Check sheet for the modelled part. Datum: model origin and axes. Units: mm. A direction names the side the tool comes from. Coordinates: 2 decimals unless noted, no trailing zeros. Write each loop counter-clockwise with the first axis right and the second up, starting at its lowest first coordinate (ties: lowest second). Pieces come first, ordered by that corner, then holes. Notation, with made-up numbers: (-27.75, 72.25) -> (29.25, 72.25) arc R13 cw to (29.25, 89.25) -> close; hole circle Ø5 at (-24.5, 18.5). An arc over 180 degrees is marked (long way). One line per item, written item: value. Start each with the question number.
1) Sectioned sample at B-B on y = 6. Enter the section's corners in (x, z), plus the area to 3 significant figures.
2) Gauge pin test, flat ends, axial feed: P1, Ø1.7, axis at x = -13.6, y = 19.26, coming from the +Z side; P2, Ø1.5, axis at y = 21.5, z = 3.5, coming from the -X side; P3, Ø8, axis at y = 16, z = 3, coming from the -X side. Record the tip position at first contact, or that the pin passes through.
3) Sectioned sample at D-D on x = 26. Enter the section's corners in (y, z).
4) Set-up check for faces 4 (the cylindrical face through (20.723, 28.746, 8.67)), 5 (the flat face through (4.81, 22.28, 1.48)): record each of +Z, -Z, +X, -X, +Y, -Y from which the full face is reachable in a straight line by a thin tool's end or side.
5) Sectioned sample at C-C on z = 4.5. Give the number of separate pieces and of enclosed holes in the cut face, plus the area to 3 significant figures.
6) Sectioned sample at A-A on x = -7.5. Enter the section's corners in (y, z).
7) Scan lines: line 1 along X through (y, z) = (30, 9.75); line 2 along Y through (x, z) = (-13, 13.25); line 3 along Y through (x, z) = (17.5, 12.75). Record each from-to range of solid material in increasing order. Write a range as [from, to].
8) Draft check along X on faces 1 (the flat face through (21.61, 7.08, 1.48)), 2 (the flat face through (-2.744, 2.805, 1.479)), 3 (the flat face through (16.56, 12.8, 1.48)). Enter one of: +X half, -X half, draft (parallel to the pull), parting line (faces both ways), or undercut.
```python
from build123d import *

# Parameters (mm, degrees)
F0_R        = 1.75
F1_DEPTH    = 3
F0_R_2      = 1.4
F2_DEPTH    = 14.5
F3_DEPTH    = 3
F4_R        = 7
F5_T1_DEPTH = 16.6306186867
F5_T3_DEPTH = 4.3681636199
F5_T5_DEPTH = 16.0958411758
F7_DEPTH    = 3


# Not quite as in the source:
# - a fillet or chamfer that OpenCascade refuses, or shapes differently, is made with other operations: its cross-section is extruded or revolved along the edge and cut away or added
# - two fillets or chamfers of one size are made in one step


with BuildPart() as f1:
    # F0 (on Top) → F1 (new body)
    with BuildSketch(Plane.XY):
        with BuildLine():
            Line((-0.4909088138, -1.2505585665), (20.7660850672, -2.35005825))
            Line((20.7660850672, -2.35005825), (25.5381567791, -2.5968895454))
            ThreePointArc((25.5381567791, -2.5968895454), (27.0513379129, -0.9141469555), (27.3799938245, 1.3248986134))
            Line((27.3799938245, 1.3248986134), (27.2720971653, 1.8240689049))
            Line((27.2720971653, 1.8240689049), (21.7261834625, 27.4815394929))
            ThreePointArc((21.7261834625, 27.4815394929), (17.3096816882, 28.8299287619), (19.4503780507, 32.9215128838))
            Line((19.4503780507, 32.9215128838), (18.5115177807, 34.0451927012))
            Line((18.5115177807, 34.0451927012), (15.1742594532, 34.2144082882))
            Line((15.1742594532, 34.2144082882), (15.9797014768, 30.8189948872))
            Line((15.9797014768, 30.8189948872), (16.4916617939, 28.6607800556))
            Line((16.4916617939, 28.6607800556), (18.135858017, 21.7295227758))
            Line((18.135858017, 21.7295227758), (18.644845427, 19.5838405017))
            Line((18.644845427, 19.5838405017), (20.2910235881, 12.6442281836))
            Line((20.2910235881, 12.6442281836), (20.8000109982, 10.4985459094))
            Line((20.8000109982, 10.4985459094), (22.4442072213, 3.5672886297))
            Line((22.4442072213, 3.5672886297), (14.8716080252, 3.8805312748))
            Line((14.8716080252, 3.8805312748), (12.8516365903, 3.9640879479))
            Line((12.8516365903, 3.9640879479), (5.2790373942, 4.2773305929))
            Line((5.2790373942, 4.2773305929), (3.2590659592, 4.360887266))
            Line((3.2590659592, 4.360887266), (0, 4.4956994243))
            Line((0, 4.4956994243), (-4.5071129665, 11.5453820412))
            Line((-4.5071129665, 11.5453820412), (-5.9023623433, 13.727724785))
            Line((-5.9023623433, 13.727724785), (-6.7908302355, 15.1173985523))
            Line((-6.7908302355, 15.1173985523), (-9.9708875905, 20.0914019161))
            Line((-9.9708875905, 20.0914019161), (-10.4149082493, 20.7859051919))
            Line((-10.4149082493, 20.7859051919), (-11.8101576261, 22.9682479357))
            Line((-11.8101576261, 22.9682479357), (-12.6478674294, 24.2785297685))
            Line((-12.6478674294, 24.2785297685), (-13.4783331305, 23.2781674713))
            Line((-13.4783331305, 23.2781674713), (-11.5363753254, 21.4427254814))
            ThreePointArc((-11.5363753254, 21.4427254814), (-12.0316990994, 16.7032264224), (-16.4766345607, 18.4209998989))
            Line((-16.4766345607, 18.4209998989), (-15.4909088138, 7.2494414335))
            Line((-15.4909088138, 7.2494414335), (-4.9353532582, 6.7494414335))
            Line((-4.9353532582, 6.7494414335), (-0.4909088138, -1.2505585665))
        make_face()
        with Locations((23.5090911862, 0.7494414335)):
            Circle(F0_R, mode=Mode.SUBTRACT)
    extrude(amount=F1_DEPTH)

    # F0 (on Top) → F2 (join)
    with BuildSketch(Plane.XY):
        with BuildLine():
            Line((-16.9909088138, 24.2494414335), (-16.4766345607, 18.4209998989))
            ThreePointArc((-16.4766345607, 18.4209998989), (-12.0316990994, 16.7032264224), (-11.5363753254, 21.4427254814))
            Line((-11.5363753254, 21.4427254814), (-13.4783331305, 23.2781674713))
            Line((-13.4783331305, 23.2781674713), (-12.6478674294, 24.2785297685))
            Line((-12.6478674294, 24.2785297685), (-11.3383288336, 25.8559736489))
            Line((-11.3383288336, 25.8559736489), (-9.782692223, 27.729862253))
            Line((-9.782692223, 27.729862253), (-8.1632279798, 29.680636341))
            Line((-8.1632279798, 29.680636341), (-6.4480341787, 31.746724331))
            Line((-6.4480341787, 31.746724331), (-4.9677388347, 33.5298583591))
            ThreePointArc((-4.9677388347, 33.5298583591), (-4.3296328325, 33.596636032), (-3.691225205, 33.6604657178))
            ThreePointArc((-3.691225205, 33.6604657178), (-2.7124843131, 33.7525453098), (-1.7331162834, 33.8376960422))
            ThreePointArc((-1.7331162834, 33.8376960422), (1.9635943301, 34.0963274062), (5.6658885292, 34.2562561568))
            ThreePointArc((5.6658885292, 34.2562561568), (6.6605332405, 34.2823712951), (7.6553394943, 34.3013612736))
            ThreePointArc((7.6553394943, 34.3013612736), (11.4153879508, 34.3087710358), (15.1742594532, 34.2144082882))
            Line((15.1742594532, 34.2144082882), (18.5115177807, 34.0451927012))
            Line((18.5115177807, 34.0451927012), (19.4503780507, 32.9215128838))
            ThreePointArc((19.4503780507, 32.9215128838), (17.3096816882, 28.8299287619), (21.7261834625, 27.4815394929))
            Line((21.7261834625, 27.4815394929), (21.7201782041, 27.5093220636))
            Line((21.7201782041, 27.5093220636), (28.8304557098, 35.6590934098))
            ThreePointArc((28.8304557098, 35.6590934098), (10.8304557098, 36.6599030898), (-7.1695442902, 35.6590934098))
            Line((-7.1695442902, 35.6590934098), (-16.9909088138, 24.2494414335))
        make_face()
        with Locations((-13.5970591864, 19.2624543916)):
            Circle(F0_R_2, mode=Mode.SUBTRACT)
        with Locations((20.077256969, 29.9877400872)):
            Circle(F0_R_2, mode=Mode.SUBTRACT)
    extrude(amount=F2_DEPTH)

    # F0 (on Top) → F3 (join)
    with BuildSketch(Plane.XY):
        with BuildLine():
            Line((-9.782692223, 27.729862253), (-11.3383288336, 25.8559736489))
            Line((-11.3383288336, 25.8559736489), (-10.6418538761, 22.9199207303))
            Line((-10.6418538761, 22.9199207303), (-11.8101576261, 22.9682479357))
            Line((-11.8101576261, 22.9682479357), (-10.4149082493, 20.7859051919))
            Line((-10.4149082493, 20.7859051919), (-10.132866466, 20.7742384561))
            Line((-10.132866466, 20.7742384561), (-9.9708875905, 20.0914019161))
            Line((-9.9708875905, 20.0914019161), (-6.7908302355, 15.1173985523))
            Line((-6.7908302355, 15.1173985523), (-8.112895031, 20.690681783))
            Line((-8.112895031, 20.690681783), (-0.540295835, 20.3774391379))
            Line((-0.540295835, 20.377439138), (1.1058823261, 13.4378268199))
            Line((1.1058823261, 13.4378268199), (-5.9023623433, 13.727724785))
            Line((-5.9023623433, 13.727724785), (-4.5071129665, 11.5453820412))
            Line((-4.5071129665, 11.5453820412), (1.6148697362, 11.2921445457))
            Line((1.6148697362, 11.2921445457), (3.2590659592, 4.360887266))
            Line((3.2590659592, 4.360887266), (5.2790373942, 4.2773305929))
            Line((5.2790373942, 4.2773305929), (3.6348411711, 11.2085878727))
            Line((3.6348411711, 11.2085878727), (11.2074403672, 10.8953452276))
            Line((11.2074403672, 10.8953452276), (12.8516365903, 3.9640879479))
            Line((12.8516365903, 3.9640879479), (14.8716080252, 3.8805312748))
            Line((14.8716080252, 3.8805312748), (13.2274118021, 10.8117885545))
            Line((13.2274118021, 10.8117885545), (20.8000109982, 10.4985459094))
            Line((20.8000109982, 10.4985459094), (20.2910235881, 12.6442281836))
            Line((20.2910235881, 12.6442281836), (12.7184243921, 12.9574708287))
            Line((12.7184243921, 12.9574708287), (11.072246231, 19.8970831467))
            Line((11.072246231, 19.8970831467), (18.644845427, 19.5838405017))
            Line((18.644845427, 19.5838405017), (18.135858017, 21.7295227758))
            Line((18.135858017, 21.7295227758), (10.5632588209, 22.0427654209))
            Line((10.5632588209, 22.0427654209), (8.9190625979, 28.9740227006))
            Line((8.9190625979, 28.9740227006), (16.4916617939, 28.6607800556))
            Line((16.4916617939, 28.6607800556), (15.9797014768, 30.8189948872))
            Line((15.9797014768, 30.8189948872), (8.4071022808, 31.1322375323))
            Line((8.4071022808, 31.1322375323), (7.6553394943, 34.3013612736))
            ThreePointArc((7.6553394943, 34.3013612736), (6.6605332405, 34.2823712951), (5.6658885292, 34.2562561568))
            Line((5.6658885292, 34.2562561568), (6.3871308458, 31.2157942054))
            Line((6.3871308458, 31.2157942054), (-1.1854683502, 31.5290368504))
            Line((-1.1854683502, 31.5290368504), (-1.7331162834, 33.8376960422))
            ThreePointArc((-1.7331162834, 33.8376960422), (-2.7124843131, 33.7525453098), (-3.691225205, 33.6604657178))
            Line((-3.691225205, 33.6604657178), (-3.2054397853, 31.6125935235))
            Line((-3.2054397853, 31.6125935235), (-6.4480341787, 31.746724331))
            Line((-6.4480341787, 31.746724331), (-8.1632279798, 29.680636341))
            Line((-8.1632279798, 29.680636341), (-2.6934794682, 29.4543786918))
            Line((-2.6934794682, 29.4543786918), (-1.0492832451, 22.5231214121))
            Line((-1.0492832451, 22.5231214121), (-8.6218824411, 22.8363640572))
            Line((-8.6218824411, 22.8363640572), (-9.782692223, 27.729862253))
        make_face()
        Polygon((1.4796756, 20.2938824649), (9.052274796, 19.9806398198), (10.6984529571, 13.0410275017), (3.1258537611, 13.3542701468), align=None, mode=Mode.SUBTRACT)
        Polygon((8.543287386, 22.126322094), (0.9706881899, 22.439564739), (-0.6735080331, 29.3708220188), (6.8990911629, 29.0575793737), align=None, mode=Mode.SUBTRACT)
    extrude(amount=F3_DEPTH)

    # F4
    f4_edges = [f1.edges().sort_by_distance(p)[0] for p in [
        (-7.169544, 35.659093, 7.25),
    ]]
    fillet(f4_edges, radius=F4_R)

    # F5: fillet of radius 3 on 3 edges, made by hand

    # F5_s2 → F5_t1 (cut)
    with BuildSketch(Plane.XY.offset(-6.8153093434)):
        with BuildLine():
            ThreePointArc((27.2309502901, -0.4600225022), (26.0778302758, -2.0046934728), (24.2228512202, -2.5288564993))
            Line((24.2228512202, -2.5288564993), (25.5381567791, -2.5968895454))
            ThreePointArc((25.5381567791, -2.5968895454), (26.5766364437, -1.6806211776), (27.2309502901, -0.4600225022))
        make_face()
    extrude(amount=F5_T1_DEPTH, mode=Mode.SUBTRACT)

    # F5_s4 → F5_t3 (cut)
    with BuildSketch(Plane.XY.offset(-0.6840818099)):
        with BuildLine():
            ThreePointArc((27.3520636944, 1.4541138391), (27.3881865873, 1.2545487843), (27.4107435182, 1.0529991394))
            ThreePointArc((27.4107435182, 1.0529991394), (27.3977458408, 1.1892177156), (27.3799938245, 1.3248986134))
            Line((27.3799938245, 1.3248986134), (27.3520636944, 1.4541138391))
        make_face()
    extrude(amount=F5_T3_DEPTH, mode=Mode.SUBTRACT)

    # F5_s6 → F5_t5 (cut)
    with BuildSketch(Plane.XY.offset(-6.5479205879)):
        with BuildLine():
            ThreePointArc((-15.7211174898, 9.8584730948), (-14.8104709381, 7.9581341855), (-12.8746740451, 7.1255145234))
            Line((-12.8746740451, 7.1255145234), (-15.4909088138, 7.2494414335))
            Line((-15.4909088138, 7.2494414335), (-15.7211174898, 9.8584730948))
        make_face()
    extrude(amount=F5_T5_DEPTH, mode=Mode.SUBTRACT)

    # F0 (on Top) → F7 (join)
    with BuildSketch(Plane.XY):
        with Locations((20.077256969, 29.9877400872)):
            Circle(F0_R_2)
        with Locations((-13.5970591864, 19.2624543916)):
            Circle(F0_R_2)
    extrude(amount=F7_DEPTH)


solid = f1.part
```
Answers:
1. outline: (-4.52, 0) -> (-0.96, 0) -> (-0.96, 3) -> (-4.52, 3) -> close; (2.87, 0) -> (4.87, 0) -> (4.87, 3) -> (2.87, 3) -> close; (12.37, 0) -> (14.37, 0) -> (14.37, 3) -> (12.37, 3) -> close; (21.87, 0) -> (26.37, 0) -> (26.37, 3) -> (21.87, 3) -> close
1. area: 36.2 mm2
2. P1: stops at z = 3
2. P2: stops at x = -16.81
2. P3: stops at x = -16.62
3. outline: (-2.06, 0) -> (7.71, 0) -> (7.71, 3) -> (-2.06, 3) -> close; (32.41, 0) -> (35.95, 0) -> (35.95, 14.5) -> (32.41, 14.5) -> close
4. face 4: +Z
4. face 5: +Z, -Z
5. separate pieces: 1
5. enclosed holes: 2
5. area: 192 mm2
6. outline: (6.87, 0) -> (18.11, 0) -> (18.11, 3) -> (6.87, 3) -> close; (20.67, 0) -> (22.79, 0) -> (22.79, 3) -> (20.67, 3) -> close; (29.65, 0) -> (34.85, 0) -> (34.85, 14.5) -> (30.48, 14.5) -> (30.48, 3) -> (29.65, 3) -> close
7. line 1: x = [-12.04, -7.9], [17.08, 18.68], [21.48, 23.89]
7. line 2: y = [16.32, 18], [20.53, 22.83], [23.85, 28.89]
7. line 3: y = [28.45, 31.52], [34.1, 36.52]
8. face 1: undercut
8. face 2: -X half
8. face 3: undercut
